Solid Edge part; units mm, degrees
sketch "Sketch1" plane through (0, 0, 0) normal (0, 0, 1) x (1, 0, 0)
  line L0 (9, 9) -> (-9, 9)
  line L1 (-9, 9) -> (-9, -9)
  line L2 (-9, -9) -> (9, -9)
  line L3 (9, -9) -> (9, 9)
extrude "Protrusion1" add sketch "Sketch1" along normal blind 8
sketch "Sketch2" plane through (0, 0, 8) normal (0, 0, 1) x (-1, 0, 0)
  circle A0 centre (0, 0) radius 5
extrude "ExtrudedProtrusion_2" add sketch "Sketch2" along normal blind 10
sketch "Sketch3" plane through (0, 0, 18) normal (0, 0, 1) x (-1, 0, 0)
  circle A0 centre (0, 0) radius 2.5
extrude "ExtrudedProtrusion_3" add sketch "Sketch3" along normal blind 35
Geometry: final body of the model. Coordinates: model frame, mm. A direction names the side the tool comes from. Round coordinates to 2 decimals unless told otherwise and drop trailing zeros. Order: outer loops, then holes, each group sorted by start corner. A loop starts at its lowest first (then second) coordinate and runs counter-clockwise, first axis right, second up. Notation, with made-up numbers: (34, 32.25) - (87, 32.25) arc R13 ccw to (87, 47.25) - close; hole circle Ø4 at (7.25, 55). An arc over 180 degrees is marked (long way). Write each question's results on one line, items separated by ' | '.
Item 1: Reachability of faces 1 (the flat face through (2, -2, 18)), 2 (the flat face through (0, 0, 0)) from +Z, -Z, +X, -X, +Y, -Y: full face, straight path, thin tool, end or side. Return the list, or none.
Completed:
face 1: +Z | face 2: -Z, +X, -X, +Y, -Y
Item 2: First-contact query: pin 1 Ø10 at (y, z) = (5, 39.5) entering from -X; pin 2 Ø6 at (x, z) = (0, 19) entering from +Y; pin 3 Ø1 at (y, z) = (2.5, 32) entering from +X. Flat tips, straight axial feed; report the tip coordinate or a pass-through.
Completed:
pin 1: x = -2.5 | pin 2: y = 5 | pin 3: x = 1.5
Item 3: Section C-C, the plane z = 11. Return the cut outline in (x, y), and give its area (3 significant figures).
Completed:
outline: circle Ø10 at (0, 0) | area: 78.5 mm^2
Item 4: Material intervals for line 1 along Y through (x, z) = (-0.25, 26); line 2 along Z through (x, y) = (-3, 5.5); line 3 along Z through (x, y) = (4.5, -0.5), sorted ascending. Write a range as [from, to].
Completed:
line 1: [-2.49, 2.49] | line 2: [0, 8] | line 3: [0, 18]
Item 5: Section D-D, the plane x = 0. Return the cut outline in (y, z).
Completed:
outline: (-9, 0) - (9, 0) - (9, 8) - (5, 8) - (5, 18) - (2.5, 18) - (2.5, 53) - (-2.5, 53) - (-2.5, 18) - (-5, 18) - (-5, 8) - (-9, 8) - close
Item 6: Section A-A, the plane x = 4. Return the cut outline in (y, z), and give its area (3 significant figures).
Completed:
outline: (-9, 0) - (9, 0) - (9, 8) - (3, 8) - (3, 18) - (-3, 18) - (-3, 8) - (-9, 8) - close | area: 204 mm^2
